Input: part model. Units: mm. Frame: model coordinates. Coordinates: 2 decimals unless noted, no trailing zeros. Write each loop counter-clockwise with the first axis right and the second up, starting at its lowest first coordinate (ties: lowest second). Pieces come first, ordered by that corner, then holes.
1) Pin query (flat end, axial travel): pin 1 Ø6 at (x, y) = (-353, 157.93) entering from +Z; pin 2 Ø1.6 at (x, z) = (358, -1.5) entering from -Y; pin 3 Ø3 at (y, z) = (-144, -1.5) entering from -X; pin 4 Ø9 at (y, z) = (-149.5, 12) entering from +X. Return the tip coordinate at first contact, or that it passes through.
2) Section query B-B (y = 69). Output: boundary loops of the cut face in (x, z).
3) Section query A-A (x = 39). Output: boundary loops of the cut face in (y, z).
4) Line query: L1, parallel to X at y = -143.85, z = 15; L2, parallel to X at y = -144.5, z = 15; L3, parallel to Y at x = -152.5, z = -2. Output: solid intervals per line, ascending.
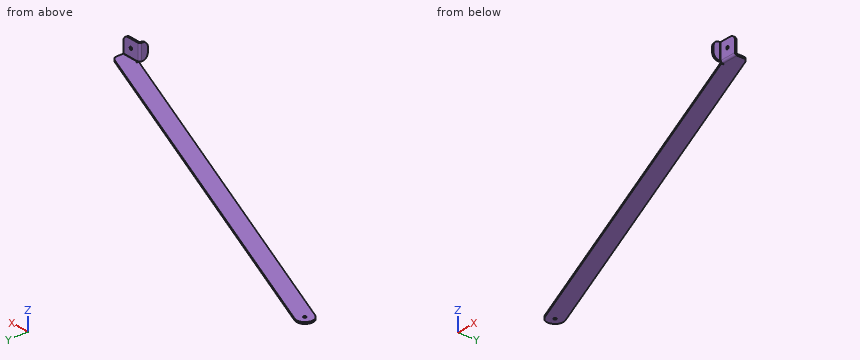
from build123d import *

# Parameters (mm, degrees)
SKETCH1_R                      = 2.55
BASE_FLANGE1_DEPTH             = 3
EDGE_FLANGE1_STRIP_W           = 14.8732
EDGE_FLANGE1_STRIP_H           = 3
EDGE_FLANGE1_STRIP_CUT_DEPTH   = 30
EDGE_FLANGE1_RELIEF_W          = 16.3732
EDGE_FLANGE1_RELIEF_H          = 1.5
EDGE_FLANGE1_RELIEF_CUT_DEPTH  = 3
EDGE_FLANGE1_DEPTH             = 30
EDGE_FLANGE2_DEPTH             = 29.2634
FILLET1_R                      = 10
F_5_1_5_1_DIAMETER_HOLE1_D     = 5.1
F_5_1_5_1_DIAMETER_HOLE1_DEPTH = 10
F_5_1_5_1_DIAMETER_HOLE1_TIP   = 1.532194579


# Sheet-metal steps are written as plain solids
with BuildPart() as part:
    # Sketch1 → Base-Flange1 (new body)
    with BuildSketch(Plane.XY):
        with BuildLine():
            Line((358.5885, -144.00735), (-358.5885, 144.00735))
            ThreePointArc((-358.5885, 144.00735), (-366.917987263, 163.516825696), (-347.408511566, 171.846312959))
            Line((-347.408511566, 171.846312959), (382.315162811, -121.207068785))
            ThreePointArc((382.315162811, -121.207068785), (386.873022561, -124.886126177), (388.5885, -130.486723104))
            Line((388.5885, -130.486723104), (388.5885, -144.00735))
            Line((388.5885, -144.00735), (358.5885, -144.00735))
        make_face()
        with Locations((-352.998505783, 157.926831479)):
            Circle(SKETCH1_R, mode=Mode.SUBTRACT)
    extrude(amount=-BASE_FLANGE1_DEPTH)

    # Edge-Flange1 strip (across the edge) → Edge-Flange1 strip cut (cut)
    with BuildSketch(Plane(origin=(358.5885, -145.40735, 0), x_dir=(0, 1, 0), z_dir=(1, 0, 0))):
        with Locations((-3.7, -1.5)):
            Rectangle(EDGE_FLANGE1_STRIP_W, EDGE_FLANGE1_STRIP_H)
    extrude(amount=EDGE_FLANGE1_STRIP_CUT_DEPTH, mode=Mode.SUBTRACT)

    # Edge-Flange1 relief (on the sheet) → Edge-Flange1 relief cut (cut)
    with BuildSketch(Plane(origin=(358.5885, -141.67075, 0), x_dir=(0, 1, 0), z_dir=(0, 0, 1))):
        with Locations((-6.6866, 0.75)):
            Rectangle(EDGE_FLANGE1_RELIEF_W, EDGE_FLANGE1_RELIEF_H)
    extrude(amount=-EDGE_FLANGE1_RELIEF_CUT_DEPTH, mode=Mode.SUBTRACT)

    # Edge-Flange1 section (across the edge) → Edge-Flange1 (add)
    with BuildSketch(Plane(origin=(358.5885, -145.40735, 0), x_dir=(0, 1, 0), z_dir=(1, 0, 0))):
        with BuildLine():
            Line((0, 0.7366), (0, 30))
            Line((0, 30), (3, 30))
            Line((3, 30), (3, 0.7366))
            ThreePointArc((3, 0.7366), (3.215745145, 0.215745145), (3.7366, 0))
            Line((3.7366, 0), (3.7366, -3))
            ThreePointArc((3.7366, -3), (1.094424801, -1.905575199), (0, 0.7366))
        make_face()
    extrude(amount=EDGE_FLANGE1_DEPTH)

    # Edge-Flange2 section (across the edge) → Edge-Flange2 (add)
    with BuildSketch(Plane(origin=(357.0519, -145.40735, 30), x_dir=(1, 0, 0), z_dir=(0, 0, -1))):
        with BuildLine():
            Line((-3, 0.7366), (-3, 12))
            Line((-3, 12), (0, 12))
            Line((0, 12), (0, 0.7366))
            ThreePointArc((0, 0.7366), (0.215745145, 0.215745145), (0.7366, 0))
            Line((0.7366, 0), (1.5366, 0))
            Line((1.5366, 0), (1.5366, -3))
            Line((1.5366, -3), (0.7366, -3))
            ThreePointArc((0.7366, -3), (-1.905575199, -1.905575199), (-3, 0.7366))
        make_face()
    extrude(amount=EDGE_FLANGE2_DEPTH)

    # Fillet1
    fillet1_edges = [part.edges().sort_by_distance(p)[0] for p in [
        (388.5885, -143.90735, 30),
        (355.5519, -157.40735, 30),
        (355.5519, -157.40735, 0.7366),
    ]]
    fillet(fillet1_edges, radius=FILLET1_R)

    # Ø5.1 (5.1) Diameter Hole1
    with Locations(Plane(origin=(0, -142.40735, 0), x_dir=(1, 0, 0), z_dir=(0, 1, 0))):
        with Locations((372.5585, -15)):
            Hole(F_5_1_5_1_DIAMETER_HOLE1_D / 2, depth=F_5_1_5_1_DIAMETER_HOLE1_DEPTH)
            with Locations((0, 0, -(F_5_1_5_1_DIAMETER_HOLE1_DEPTH + F_5_1_5_1_DIAMETER_HOLE1_TIP / 2))):  # 118° drill point
                Cone(0, F_5_1_5_1_DIAMETER_HOLE1_D / 2, F_5_1_5_1_DIAMETER_HOLE1_TIP, mode=Mode.SUBTRACT)


solid = part.part
Answer:
1. pin 1: stops at z = 0
1. pin 2: stops at y = -145
1. pin 3: stops at x = 354.84
1. pin 4: stops at x = 388.59
2. outline: (-171.81, -3) - (-91.31, -3) - (-91.31, 0) - (-171.81, 0) - close
3. outline: (-15.66, -3) - (16.67, -3) - (16.67, 0) - (-15.66, 0) - close
4. L1: x = 354.84 to 370.01, 375.11 to 388.59
4. L2: x = 354.43 to 370.01, 375.11 to 388.59
4. L3: y = 61.24 to 93.57
